The listing builds one solid part. Answer for the finished solid, in the listing's coordinates (mm). A direction names the side the tool comes from. Round coordinates to 2 decimals unless told otherwise and drop trailing zeros. Write each loop counter-clockwise with the first axis right and the second up, starting at its lowest first coordinate (ties: lowest second). Pieces come first, ordered by that corner, then holes. Notation, with made-up numbers: (-30, 26) - (-26, 26) arc R20 ccw to (-26, 46) - close; hole circle Ø9 at (26, 60). An arc over 180 degrees is marked (long way). Use a Markdown table: item, result. Add a question column.
1) A tool of negligible diameter and unlimited length cuts with its end or side. For faces 5 (the flat face through (14.65, 0, 23)), 6 (the cylindrical face through (-13.79, 29.35, 23.62)), 7 (the cylindrical face through (13.79, -29.35, 23.62)), 8 (the flat face through (0, -30.25, 23)), 9 (the flat face through (-4.9, -14, -6)), from which of +Z, -Z, +X, -X, +Y, -Y can it reach the whole face along a straight path? Write none if from no direction.
2) A cutting plane is placed at C-C (z = 27). Give the vertices of the cut face in (x, y), then the cut area to 3 significant figures.
3) A cutting plane is placed at B-B (y = 21). Give the vertices of the cut face in (x, z), then the cut area to 3 significant figures.
4) Determine the mould class of faces 1 (the cylindrical face through (13.75, 29.39, 23.62)), 2 (the flat face through (0, -25.87, -5)), 3 (the flat face through (0, -25.05, -5)), 4 (the flat face through (0, -20.25, -1)) for opening direction Y: +Y half, -Y half, draft (parallel to the pull), parting line (faces both ways), or undercut.
5) A cutting plane is placed at A-A (x = 0). Give the vertices of the cut face in (y, z), then the cut area to 3 significant figures.
6) Each of these flat-tipped pins is pushed along its axis until it touches: P1, Ø4, axis at x = -3, z = 30.5, coming from the +Y side; P2, Ø6, axis at x = -5.5, y = -30.5, coming from the -Z side; P3, Ø3, axis at y = -13.5, z = -6, coming from the +X side. Where does it stop, or does it pass through?
7) Find the intervals of material crossed by probe 1 along Y at (x, z) = (0, 44); probe 2 along Z at (x, y) = (12, 6); probe 3 along Y at (x, z) = (11.5, 11), in increasing order. Write a range as from..to.
8) A cutting plane is placed at D-D (y = 36). Give the vertices of the cut face in (x, z), then the cut area to 3 significant figures.
```python
from build123d import *

# Parameters (mm, degrees)
SKETCH1_W           = 29.3
SKETCH1_H           = 60.5
BOSS_EXTRUDE1_DEPTH = 43.67
SKETCH2_R           = 1.6
BOSS_EXTRUDE2_DEPTH = 2.5
FILLET1_R           = 3
SKETCH3_W           = 21
SKETCH3_H           = 13
BOSS_EXTRUDE3_DEPTH = 2
SKETCH4_W           = 0.82
SKETCH4_H           = 6.4
BOSS_EXTRUDE4_DEPTH = 7.85
SKETCH5_W           = 6.4
SKETCH5_H           = 0.82
BOSS_EXTRUDE5_DEPTH = 9.85
CHAMFER1_SIZE       = 1


with BuildPart() as part:
    # Sketch1 → Boss-Extrude1 (new body)
    with BuildSketch(Plane.XY):
        Rectangle(SKETCH1_W, SKETCH1_H)
    extrude(amount=BOSS_EXTRUDE1_DEPTH)

    # Sketch2 → Boss-Extrude2 (add)
    with BuildSketch(Plane.XY.offset(43.67)):
        with BuildLine():
            Line((-16, 32), (-2.62619365, 40.254774602))
            ThreePointArc((-2.62619365, 40.254774602), (0, 41), (2.62619365, 40.254774602))
            Line((2.62619365, 40.254774602), (16, 32))
            Line((16, 32), (16, -32))
            Line((16, -32), (2.62619365, -40.254774602))
            ThreePointArc((2.62619365, -40.254774602), (0, -41), (-2.62619365, -40.254774602))
            Line((-2.62619365, -40.254774602), (-16, -32))
            Line((-16, -32), (-16, 32))
        make_face()
        with Locations((0, 36)):
            Circle(SKETCH2_R, mode=Mode.SUBTRACT)
        with Locations(Location((0, -36, 0), (0, 0, 180))):
            Circle(SKETCH2_R, mode=Mode.SUBTRACT)
    extrude(amount=BOSS_EXTRUDE2_DEPTH)

    # Fillet1
    fillet1_edges = [part.edges().sort_by_distance(p)[0] for p in [
        (0, -30.25, 0),
        (-14.65, 0, 0),
        (0, 30.25, 0),
        (14.65, 0, 0),
        (14.65, -30.25, 21.835),
        (-14.65, -30.25, 21.835),
        (-14.65, 30.25, 21.835),
        (14.65, 30.25, 21.835),
    ]]
    fillet(fillet1_edges, radius=FILLET1_R)

    # Sketch3 → Boss-Extrude3 (add)
    with BuildSketch(Plane(origin=(0, 0, 0), x_dir=(-1, 0, 0), z_dir=(0, 0, -1))):
        with Locations((0, -13.75)):
            Rectangle(SKETCH3_W, SKETCH3_H)
    extrude(amount=BOSS_EXTRUDE3_DEPTH)

    # Sketch4 → Boss-Extrude4 (add)
    with BuildSketch(Plane(origin=(0, 0, -2), x_dir=(-1, 0, 0), z_dir=(0, 0, -1))):
        with Locations((-5.31, -13.75)):
            Rectangle(SKETCH4_W, SKETCH4_H)
        with Locations((5.31, -13.75)):
            Rectangle(SKETCH4_W, SKETCH4_H)
    extrude(amount=BOSS_EXTRUDE4_DEPTH)

    # Sketch5 → Boss-Extrude5 (add)
    with BuildSketch(Plane(origin=(0, 0, 0), x_dir=(-1, 0, 0), z_dir=(0, 0, -1))):
        with Locations((0, -25.46)):
            Rectangle(SKETCH5_W, SKETCH5_H)
    extrude(amount=BOSS_EXTRUDE5_DEPTH)

    # Chamfer1
    chamfer1_edges = [part.edges().sort_by_distance(p)[0] for p in [
        (-5.31, -16.95, -9.85),
        (-5.31, -10.55, -9.85),
        (-3.2, -25.46, -9.85),
        (3.2, -25.46, -9.85),
        (5.31, -16.95, -9.85),
        (5.31, -10.55, -9.85),
    ]]
    chamfer(chamfer1_edges, length=CHAMFER1_SIZE)


solid = part.part
```
Entries:
| question | item | result |
|---|---|---|
| 1 | face 5 | -Z, +X, +Y, -Y |
| 1 | face 6 | -Z, -X, +Y |
| 1 | face 7 | -Z, +X, -Y |
| 1 | face 8 | -Z, +X, -X, -Y |
| 1 | face 9 | -Z, +Y, -Y |
| 2 | outline | (-14.65, -27.25) arc R3 ccw to (-11.65, -30.25) - (11.65, -30.25) arc R3 ccw to (14.65, -27.25) - (14.65, 27.25) arc R3 ccw to (11.65, 30.25) - (-11.65, 30.25) arc R3 ccw to (-14.65, 27.25) - close |
| 2 | area | 1,760 mm² |
| 3 | outline | (-16, 43.67) - (-14.65, 43.67) - (-14.65, 3) arc R3 ccw to (-11.65, 0) - (11.65, 0) arc R3 ccw to (14.65, 3) - (14.65, 43.67) - (16, 43.67) - (16, 46.17) - (-16, 46.17) - close |
| 3 | area | 1,360 mm² |
| 4 | face 1 | +Y half |
| 4 | face 2 | -Y half |
| 4 | face 3 | undercut |
| 4 | face 4 | undercut |
| 5 | outline | (-41, 43.67) - (-37.6, 43.67) - (-37.6, 46.17) - (-41, 46.17) - close; (-34.4, 43.67) - (-30.25, 43.67) - (-30.25, 3) arc R3 ccw to (-27.25, 0) - (-25.87, 0) - (-25.87, -9.85) - (-25.05, -9.85) - (-25.05, 0) - (-20.25, 0) - (-20.25, -2) - (-7.25, -2) - (-7.25, 0) - (27.25, 0) arc R3 ccw to (30.25, 3) - (30.25, 43.67) - (34.4, 43.67) - (34.4, 46.17) - (-34.4, 46.17) - close; (37.6, 43.67) - (41, 43.67) - (41, 46.17) - (37.6, 46.17) - close |
| 5 | area | 2,860 mm² |
| 6 | P1 | stops at y = 30.25 |
| 6 | P2 | stops at z = 0.01 |
| 6 | P3 | stops at x = 5.72 |
| 7 | probe 1 | y = -41..-37.6, -34.4..34.4, 37.6..41 |
| 7 | probe 2 | z = 0.02..46.17 |
| 7 | probe 3 | y = -30.25..30.25 |
| 8 | outline | (-9.52, 43.67) - (-1.6, 43.67) - (-1.6, 46.17) - (-9.52, 46.17) - close; (1.6, 43.67) - (9.52, 43.67) - (9.52, 46.17) - (1.6, 46.17) - close |
| 8 | area | 39.6 mm² |
